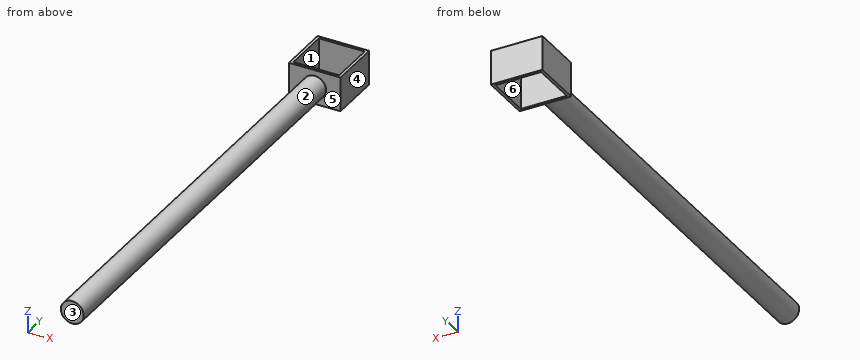
```python
from build123d import *

# Parameters (mm, degrees)
SKETCH1_W           = 57.15
SKETCH1_H           = 57.15
SKETCH1_W_2         = 50.8
SKETCH1_H_2         = 50.8
BOSS_EXTRUDE1_DEPTH = 38.1
SKETCH4_R           = 12.7
BOSS_EXTRUDE2_DEPTH = 482.6


with BuildPart() as part:
    # Sketch1 → Boss-Extrude1 (new body)
    with BuildSketch(Plane.XY):
        Rectangle(SKETCH1_W, SKETCH1_H)
        Rectangle(SKETCH1_W_2, SKETCH1_H_2, mode=Mode.SUBTRACT)
    extrude(amount=BOSS_EXTRUDE1_DEPTH)

    # Sketch4 → Boss-Extrude2 (add)
    with BuildSketch(Plane(origin=(0, -27.94, 0), x_dir=(1, 0, 0), z_dir=(0, 1, 0))):
        with Locations(Location((0, -19.05, 0), (0, 0, 270))):
            Circle(SKETCH4_R)
    extrude(amount=-BOSS_EXTRUDE2_DEPTH)


solid = part.part
```
Geometry: final body of the model. Coordinates: model frame, mm. Face numbers are marked on the shaded views. A direction names the side the tool comes from. Round coordinates to 2 decimals unless told otherwise and drop trailing zeros. Order: outer loops, then holes, each group sorted by start corner. A loop starts at its lowest first (then second) coordinate and runs counter-clockwise, first axis right, second up. Notation, with made-up numbers: (-22.75, 78.5) -> (-1.75, 78.5) arc R18 cw to (-1.75, 95.5) -> close; hole circle Ø6 at (32.5, 18). An arc over 180 degrees is marked (long way). Use one line per item in the form item = value.
(1) First-contact query: pin 1 Ø6 at (x, z) = (19, 30) entering from -Y (3 decimals); pin 2 Ø12 at (y, z) = (-47.5, 5.5) entering from -X; pin 3 Ø1 at (x, y) = (-0.5, -434.5) entering from +Z. Flat tips, straight axial feed; report the tip coordinate or a pass-through.
Results list:
pin_1 = -28.575
pin_2 = -10.21
pin_3 = 31.75
(2) Section C-C on y = -312. Return loops of the section in (x, z).
Results list:
outline = circle Ø25.4 at (0, 19.05)
(3) Access query for the marked faces 4, 5 and 6. Directions: +Z, -Z, +X, -X, +Y, -Y. A direction counts if a zero-diameter tool reaches every point of the face in a straight line with its end or side. Return the directions, or none.
Results list:
face_4 = +Z, -Z, +X, +Y, -Y
face_5 = -Y
face_6 = +Z, -Z
(4) Section B-B on z = 19.05. Return loops of the section in (x, y) (3 decimals).
Results list:
outline = (-28.575, -28.575) -> (-12.7, -28.575) -> (-12.7, -510.54) -> (12.7, -510.54) -> (12.7, -28.575) -> (28.575, -28.575) -> (28.575, 28.575) -> (-28.575, 28.575) -> close; hole (-25.4, -25.4) -> (25.4, -25.4) -> (25.4, 25.4) -> (-25.4, 25.4) -> close
(5) Ray query, probe 1 along Y at (x, z) = (15.5, 22) (3 decimals); probe 2 along Y at (x, z) = (10, 19) (3 decimals); probe 3 along Z at (x, y) = (1.5, -323). Return the intervals inside material, ascending. Write a range as [from, to].
Results list:
probe_1 = [-28.575, -25.4], [25.4, 28.575]
probe_2 = [-510.54, -25.4], [25.4, 28.575]
probe_3 = [6.44, 31.66]
(6) Draft query along Y for the marked faces 1, 2 and 3. Return one class per face: pulls with the +Y half, pulls with the -Y half, needs draft (parallel to the pull), parting line crosses it, or undercut.
Results list:
face_1 = undercut
face_2 = needs draft
face_3 = pulls with the -Y half
(7) Section A-A on x = 0. Return loops of the section in (y, z) (3 decimals).
Results list:
outline = (-510.54, 6.35) -> (-28.575, 6.35) -> (-28.575, 0) -> (-25.4, 0) -> (-25.4, 38.1) -> (-28.575, 38.1) -> (-28.575, 31.75) -> (-510.54, 31.75) -> close; (25.4, 0) -> (28.575, 0) -> (28.575, 38.1) -> (25.4, 38.1) -> close
